from build123d import *

# Parameters (mm, degrees)
BOSS_EXTRUDE1_DEPTH = 25
SKETCH16_W          = 33.4
SKETCH16_H          = 12.9
CUT_EXTRUDE10_DEPTH = 4.5
SKETCH19_R          = 20
CUT_EXTRUDE14_DEPTH = 7.55
SKETCH17_W          = 23.6
SKETCH17_H          = 12.9
CUT_EXTRUDE11_DEPTH = 177.45821035
CUT_EXTRUDE13_DEPTH = 6.45
SKETCH20_W          = 33.4
SKETCH20_H          = 12.9
CUT_EXTRUDE15_DEPTH = 176.655202029
SKETCH21_R          = 1.1
CUT_EXTRUDE16_DEPTH = 177.45821035
SKETCH22_R          = 2
CUT_EXTRUDE17_DEPTH = 17.45
SKETCH23_W          = 162.562335495
SKETCH23_H          = 86.576971135
CUT_EXTRUDE18_DEPTH = 177.45821035
CUT_EXTRUDE19_DEPTH = 177.45821035
SKETCH26_W          = 6.440152625
SKETCH26_H          = 21.054345118
CUT_EXTRUDE20_DEPTH = 175.458005773


with BuildPart() as part:
    # Sketch1 → Boss-Extrude1 (new body)
    with BuildSketch(Plane.XY):
        with BuildLine():
            ThreePointArc((172.5, 0), (152.823244805, 26.363741023), (121.951138857, 15))
            Line((121.951138857, 15), (145, 15))
            Line((145, 15), (145, -15))
            Line((145, -15), (121.951138857, -15))
            ThreePointArc((121.951138857, -15), (152.823244805, -26.363741023), (172.5, 0))
        make_face()
        with BuildLine():
            Line((145, 15), (121.951138857, 15))
            ThreePointArc((121.951138857, 15), (117.5, 0), (121.951138857, -15))
            Line((121.951138857, -15), (145, -15))
            Line((145, -15), (145, 15))
        make_face()
        with BuildLine():
            Line((121.951138857, 15), (23.048861143, 15))
            ThreePointArc((23.048861143, 15), (26.363741023, 7.823244805), (27.5, 0))
            ThreePointArc((27.5, 0), (26.363741023, -7.823244805), (23.048861143, -15))
            Line((23.048861143, -15), (121.951138857, -15))
            ThreePointArc((121.951138857, -15), (117.5, 0), (121.951138857, 15))
        make_face()
        with BuildLine():
            ThreePointArc((13.228756555, -15), (-20, 0), (13.228756555, 15))
            Line((13.228756555, 15), (23.048861143, 15))
            ThreePointArc((23.048861143, 15), (-27.5, 0), (23.048861143, -15))
            Line((23.048861143, -15), (13.228756555, -15))
        make_face()
        with BuildLine():
            Line((23.048861143, 15), (13.228756555, 15))
            ThreePointArc((13.228756555, 15), (18.228756555, 8.228756555), (20, 0))
            ThreePointArc((20, 0), (18.228756555, -8.228756555), (13.228756555, -15))
            Line((13.228756555, -15), (23.048861143, -15))
            ThreePointArc((23.048861143, -15), (26.363741023, -7.823244805), (27.5, 0))
            ThreePointArc((27.5, 0), (26.363741023, 7.823244805), (23.048861143, 15))
        make_face()
        with BuildLine():
            Line((0, -15), (0, 15))
            Line((0, 15), (13.228756555, 15))
            ThreePointArc((13.228756555, 15), (-20, 0), (13.228756555, -15))
            Line((13.228756555, -15), (0, -15))
        make_face()
        with BuildLine():
            Line((13.228756555, 15), (0, 15))
            Line((0, 15), (0, -15))
            Line((0, -15), (13.228756555, -15))
            ThreePointArc((13.228756555, -15), (18.228756555, -8.228756555), (20, 0))
            ThreePointArc((20, 0), (18.228756555, 8.228756555), (13.228756555, 15))
        make_face()
    extrude(amount=BOSS_EXTRUDE1_DEPTH)

    # Sketch16 → Cut-Extrude10 (cut)
    with BuildSketch(Plane(origin=(0, 0, 0), x_dir=(-1, 0, 0), z_dir=(0, 0, -1))):
        with Locations((-150.21934279, 0)):
            Rectangle(SKETCH16_W, SKETCH16_H)
    extrude(amount=-CUT_EXTRUDE10_DEPTH, mode=Mode.SUBTRACT)

    # Sketch19 → Cut-Extrude14 (cut)
    with BuildSketch(Plane(origin=(0, 0, 0), x_dir=(-1, 0, 0), z_dir=(0, 0, -1))):
        Circle(SKETCH19_R)
    extrude(amount=-CUT_EXTRUDE14_DEPTH, mode=Mode.SUBTRACT)

    # Sketch17 → Cut-Extrude11 (cut, through all)
    with BuildSketch(Plane(origin=(0, 0, 0), x_dir=(-1, 0, 0), z_dir=(0, 0, -1))):
        with Locations((-150.21934279, 0)):
            Rectangle(SKETCH17_W, SKETCH17_H)
    extrude(amount=-CUT_EXTRUDE11_DEPTH, mode=Mode.SUBTRACT)

    # Sketch18 → Cut-Extrude13 (cut, symmetric)
    with BuildSketch(Plane(origin=(0, 0, 0), x_dir=(-1, 0, 0), z_dir=(0, -1, 0))):
        Polygon((-138.41934279, -15), (-138.41934279, -25), (-122.41934279, -25), (-122.41934279, -22.5), align=None)
    extrude(amount=CUT_EXTRUDE13_DEPTH, both=True, mode=Mode.SUBTRACT)

    # Sketch20 → Cut-Extrude15 (cut, through all)
    with BuildSketch(Plane(origin=(0, 0, 6.5), x_dir=(-1, 0, 0), z_dir=(0, 0, -1))):
        with Locations((-150.21934279, 0)):
            Rectangle(SKETCH20_W, SKETCH20_H)
    extrude(amount=-CUT_EXTRUDE15_DEPTH, mode=Mode.SUBTRACT)

    # Sketch21 → Cut-Extrude16 (cut, through all)
    with BuildSketch(Plane(origin=(0, 0, 0), x_dir=(-1, 0, 0), z_dir=(0, 0, -1))):
        with Locations((-163.75, 0)):
            Circle(SKETCH21_R)
        with Locations((-136.75, 0)):
            Circle(SKETCH21_R)
    extrude(amount=-CUT_EXTRUDE16_DEPTH, mode=Mode.SUBTRACT)

    # Sketch22 → Cut-Extrude17 (cut)
    with BuildSketch(Plane.XY.offset(25)):
        Circle(SKETCH22_R)
    extrude(amount=-CUT_EXTRUDE17_DEPTH, mode=Mode.SUBTRACT)

    # Sketch23 → Cut-Extrude18 (cut, through all)
    with BuildSketch(Plane(origin=(0, 0, 0), x_dir=(-1, 0, 0), z_dir=(0, 0, -1))):
        with Locations((-51.54910521, 1.570557299)):
            Rectangle(SKETCH23_W, SKETCH23_H)
    extrude(amount=-CUT_EXTRUDE18_DEPTH, mode=Mode.SUBTRACT)

    # Sketch24 → Cut-Extrude19 (cut, through all)
    with BuildSketch(Plane(origin=(0, 0, 0), x_dir=(-1, 0, 0), z_dir=(0, 0, -1))):
        with BuildLine():
            Line((-167.786941529, -7.371958929), (-171.493475075, -7.371958929))
            ThreePointArc((-171.493475075, -7.371958929), (-156.225736685, -25.104438569), (-132.830272958, -24.66065173))
            Line((-132.830272958, -24.66065173), (-132.830272958, -7.371958929))
            Line((-132.830272958, -7.371958929), (-167.786941529, -7.371958929))
        make_face()
        with BuildLine():
            Line((-185.462542345, -7.371958929), (-172.088300957, -7.371958929))
            Line((-172.088300957, -7.371958929), (-171.493475075, -7.371958929))
            ThreePointArc((-171.493475075, -7.371958929), (-172.499951334, -0.051736146), (-171.521025432, 7.272221809))
            Line((-171.521025432, 7.272221809), (-172.314497195, 7.272221809))
            Line((-172.314497195, 7.272221809), (-185.462542345, 7.272221809))
            Line((-185.462542345, 7.272221809), (-185.462542345, -7.371958929))
        make_face()
        with BuildLine():
            ThreePointArc((-132.830272958, 24.66065173), (-156.272946161, 25.083275003), (-171.521025432, 7.272221809))
            Line((-171.521025432, 7.272221809), (-167.786941529, 7.272221809))
            Line((-167.786941529, 7.272221809), (-132.830272958, 7.272221809))
            Line((-132.830272958, 7.272221809), (-132.830272958, 24.66065173))
        make_face()
    extrude(amount=-CUT_EXTRUDE19_DEPTH, mode=Mode.SUBTRACT)

    # Sketch26 → Cut-Extrude20 (cut, through all)
    with BuildSketch(Plane(origin=(0, 0, 0), x_dir=(-1, 0, 0), z_dir=(0, 0, -1))):
        with Locations((-171.097089858, -0.597985902)):
            Rectangle(SKETCH26_W, SKETCH26_H)
    extrude(amount=-CUT_EXTRUDE20_DEPTH, mode=Mode.SUBTRACT)


solid = part.part
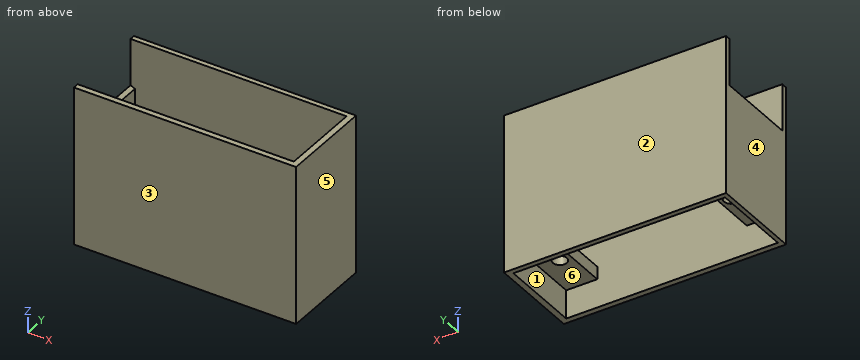
Verification items for the finished model (mm, model axes). Face numbers are marked on the shaded views. A direction names the side the tool comes from. Coordinates: 2 decimals unless noted, no trailing zeros. Order: outer loops, then holes, each group sorted by start corner. A loop starts at its lowest first (then second) coordinate and runs counter-clockwise, first axis right, second up. Notation, with made-up numbers: (-9, 51) -> (0, 51) arc R17 ccw to (0, 79) -> close; hole circle Ø4 at (20, -20.5). An arc over 180 degrees is marked (long way). Put each result on its own line as item: value. Start each with the question number.
1. Cross-section at D-D, the plane y = -4.5. Record the boundary of the cut face in (x, z).
2. Cross-section at C-C, the plane z = 7.5. Record the boundary of the cut face in (x, y), then the cut area to 3 significant figures.
3. Cross-section at A-A, the plane x = 157. Record the boundary of the cut face in (y, z), then the cut area to 3 significant figures.
4. Material ranges on L1, parallel to X at y = 0.25, z = 10; L2, parallel to Y at x = 146, z = 20.25; L3, parallel to Z at x = 164, y = 4.5, recorded low to high. Write a range as [from, to].
5. Mould release check, pull along X, two halves, no side actions. Record for the marked faces 3, 4, 5 and 6: released by +X, released by -X, zero draft, split by the parting line, or undercut.
6. Access from +Z, -Z, +X, -X, +Y, -Y to the whole of each face (thin tool, end or side, straight path). Record for the marked faces 1 and 2.
7. Cross-section at B-B, the plane y = 0. Record the boundary of the cut face in (x, z), then the cut area to 3 significant figures.
8. Go/stop test with flat-tipped pins: pin 1 Ø4 at (x, y) = (137, -3) entering from +Z; pin 2 Ø4 at (x, y) = (164.5, -1.5) entering from -Z. Record where each tip stops, or that it passes through.
Computed:
1. outline: (132.83, 0) -> (133.52, 0) -> (133.52, 4.5) -> (138.42, 4.5) -> (138.42, 6.5) -> (133.52, 6.5) -> (133.52, 17.3) -> (132.83, 17.62) -> close; (162.02, 4.5) -> (166.92, 4.5) -> (166.92, 0) -> (167.88, 0) -> (167.88, 25) -> (166.92, 25) -> (166.92, 6.5) -> (162.02, 6.5) -> close
2. outline: (132.83, -7.37) -> (167.88, -7.37) -> (167.88, 7.27) -> (132.83, 7.27) -> close; hole (133.52, -6.45) -> (166.92, -6.45) -> (166.92, 6.45) -> (133.52, 6.45) -> close
2. area: 82.4 mm2
3. outline: (-7.37, 0) -> (-6.45, 0) -> (-6.45, 25) -> (-7.37, 25) -> close; (6.45, 0) -> (7.27, 0) -> (7.27, 25) -> (6.45, 25) -> close
3. area: 43.6 mm2
4. L1: [132.83, 133.52], [166.92, 167.88]
4. L2: [-7.37, -6.45], [6.45, 7.27]
4. L3: [4.5, 6.5]
5. face 3: zero draft
5. face 4: released by -X
5. face 5: released by +X
5. face 6: undercut
6. face 1: -Z
6. face 2: +Z, -Z, +X, -X, +Y
7. outline: (132.83, 0) -> (133.52, 0) -> (133.52, 4.5) -> (135.65, 4.5) -> (135.65, 6.5) -> (133.52, 6.5) -> (133.52, 17.3) -> (132.83, 17.62) -> close; (137.85, 4.5) -> (138.42, 4.5) -> (138.42, 6.5) -> (137.85, 6.5) -> close; (162.02, 4.5) -> (162.65, 4.5) -> (162.65, 6.5) -> (162.02, 6.5) -> close; (164.85, 4.5) -> (166.92, 4.5) -> (166.92, 0) -> (167.88, 0) -> (167.88, 25) -> (166.92, 25) -> (166.92, 6.5) -> (164.85, 6.5) -> close
7. area: 46.8 mm2
8. pin 1: z = 6.5
8. pin 2: z = 4.5
